Geometry: final body of the model. Coordinates: model frame, mm. Face numbers are marked on the shaded views. Round coordinates to 2 decimals unless told otherwise and drop trailing zeros. Write each loop counter-clockwise with the first axis right and the second up, starting at its lowest first coordinate (ties: lowest second). Pieces come first, ordered by that corner, then holes. Notation, with made-up numbers: (35, 57) -> (65, 57) arc R30 cw to (65, 91) -> close; hole circle Ø3 at (11.5, 85). An arc over 180 degrees is marked (long way). Use one line per item in the form item = value. Start each with the question number.
1. Pin query (flat end, axial travel): pin 1 Ø6 at (y, z) = (-3, -6.5) entering from +X; pin 2 Ø4 at (y, z) = (-2, 15.5) entering from -X; pin 3 Ø3 at (x, z) = (-0.5, 15.5) entering from -Y. Return the tip coordinate at first contact, or that it passes through.
2. Cut plane A-A, the plane z = 13. Return the cut outline in (x, y).
3. Line query: L1, parallel to Y at x = -4, z = -12; L2, parallel to Y at x = 0, z = 18.5; L3, parallel to X at y = 3.5, z = -4.5. Output: solid intervals per line, ascending.
4. Draft query along X for the marked faces 1 and 2. Return one class per face: pulls with the +X half, pulls with the -X half, needs draft (parallel to the pull), parting line crosses it, or undercut.
5. Cut plane B-B, the plane z = -10. Return the cut outline in (x, y).
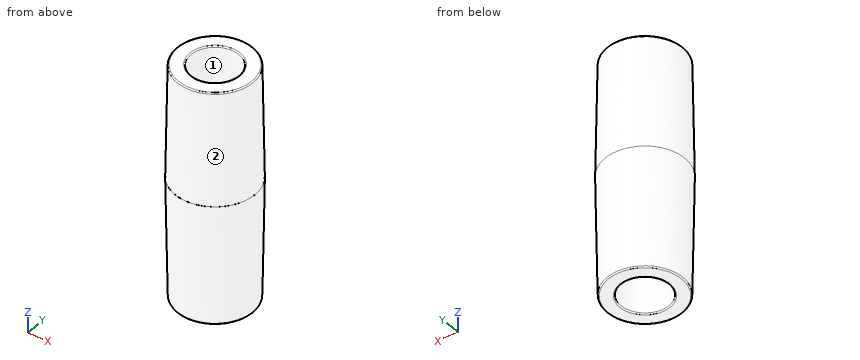
```python
from build123d import *

# Parameters (mm, degrees)
FILLET1_R = 0.254


with BuildPart() as part:
    # Sketch1 → Revolve1 (revolve)
    with BuildSketch(Plane.XZ):
        Polygon((5.047062695, 23.876), (4.8387, 0), (4.8514, 0), (5.073062442, -25.4), (7.976741351, -25.4), (8.4201, 0), (8.4074, 0), (7.99064287, 23.876), align=None)
    revolve(axis=Axis((0, 0, 23.867968573), (0, 0, -1)))

    # Fillet1
    fillet1_edges = [part.edges().sort_by_distance(p)[0] for p in [
        (-7.99064287, 0, 23.876),
        (-7.976741351, 0, -25.4),
        (-5.073062442, 0, -25.4),
        (-5.047062695, 0, 23.876),
    ]]
    fillet(fillet1_edges, radius=FILLET1_R)


solid = part.part
```
Outcome:
q1.pin_1 = 8.32
q1.pin_2 = -8.15
q1.pin_3 = -8.16
q2.outline = circle Ø16.36 at (0, 0); hole circle Ø9.9 at (0, 0)
q3.L1 = -7.17 to -2.93, 2.93 to 7.17
q3.L2 = -8.08 to -5, 5 to 8.08
q3.L3 = -7.57 to -3.42, 3.42 to 7.57
q4.face_1 = undercut
q4.face_2 = parting line crosses it
q5.outline = circle Ø16.49 at (0, 0); hole circle Ø9.88 at (0, 0)
